Source: CAD feature listing. Evaluate the final solid. Frame: model axes, mm. Face numbers are marked on the shaded views. A direction names the side the tool comes from. Coordinates: 2 decimals unless noted, no trailing zeros. Loops run counter-clockwise (first coordinate to the right, second up) from the corner with the lowest first, then second, coordinate; pieces in that order, holes last. Notation, with made-up numbers: (3.25, 9.25) -> (48.25, 9.25) arc R24 ccw to (48.25, 34.25) -> close; hole circle Ø7 at (-4, -30). An arc over 180 degrees is marked (long way). Answer as a JSON object with one key per item and string values. Group by question number.
Autodesk Inventor part; units mm, degrees
ref_plane "YZ Plane" through (0, 0, 0) normal (1, 0, 0) x (0, 1, 0)
ref_plane "XZ Plane" through (0, 0, 0) normal (0, 1, 0) x (-1, 0, 0)
ref_plane "XY Plane" through (0, 0, 0) normal (0, 0, 1) x (1, 0, 0)
sketch "Sketch4" plane through (0, 0, 0) normal (0, 0, 1) x (1, 0, 0)
  line L0 (0, 0) -> (44.9009, -44.9017) construction
  line L1 (44.9009, -44.9017) -> (89.8017, 0) construction
  line L2 (89.8017, 0) -> (0, 0) construction
  circle A0 centre (0, 0) radius 63.5 construction
  line L3 (40.1856, -49.1667) -> (14.1078, -23.0884)
  line L4 (23.0881, -14.1082) -> (49.166, -40.1866)
  arc A1 (23.0881, -14.1082) -> (14.1078, -23.0884) centre (18.5979, -18.5983) ccw
  arc A2 (56.3508, 29.2718) -> (56.3508, -29.2718) centre (89.8017, 0) ccw
  arc A3 (49.166, -40.1866) -> (56.3508, -29.2718) centre (0, 0) ccw
  arc A4 (56.3508, 29.2718) -> (49.166, 40.1866) centre (0, 0) ccw
  line L5 (49.166, 40.1866) -> (56.3508, 29.2718) construction
  line L6 (56.3508, -29.2718) -> (49.166, -40.1866) construction
  line L7 (0, 0) -> (44.9017, 44.9009) construction
  line L8 (44.9017, 44.9009) -> (0, 89.8017) construction
  line L9 (0, 89.8017) -> (0, 0) construction
  circle A5 centre (0, 0) radius 63.5 construction
  line L10 (49.166, 40.1866) -> (23.0884, 14.1078)
  line L11 (14.1082, 23.0881) -> (40.1866, 49.166)
  arc A6 (14.1082, 23.0881) -> (23.0884, 14.1078) centre (18.5983, 18.5979) ccw
  arc A7 (-29.2718, 56.3508) -> (29.2718, 56.3508) centre (0, 89.8017) ccw
  arc A8 (40.1866, 49.166) -> (29.2718, 56.3508) centre (0, 0) ccw
  arc A9 (-29.2718, 56.3508) -> (-40.1856, 49.1667) centre (0, 0) ccw
  line L12 (-40.1856, 49.1667) -> (-29.2718, 56.3508) construction
  line L13 (29.2718, 56.3508) -> (40.1866, 49.166) construction
  line L14 (0, 0) -> (-44.9008, 44.9017) construction
  line L15 (-44.9008, 44.9017) -> (-89.8017, 0) construction
  line L16 (-89.8017, 0) -> (0, 0) construction
  circle A10 centre (0, 0) radius 63.5 construction
  line L17 (-40.1856, 49.1667) -> (-14.1078, 23.0884)
  line L18 (-23.0881, 14.1082) -> (-49.166, 40.1866)
  arc A11 (-23.0881, 14.1082) -> (-14.1078, 23.0884) centre (-18.5979, 18.5983) ccw
  arc A12 (-56.3508, -29.2718) -> (-56.3508, 29.2718) centre (-89.8017, 0) ccw
  arc A13 (-49.166, 40.1866) -> (-56.3508, 29.2718) centre (0, 0) ccw
  arc A14 (-56.3508, -29.2718) -> (-49.1667, -40.1856) centre (0, 0) ccw
  line L19 (-49.1667, -40.1856) -> (-56.3508, -29.2718) construction
  line L20 (-56.3508, 29.2718) -> (-49.166, 40.1866) construction
  line L21 (0, 0) -> (-44.9017, -44.9008) construction
  line L22 (-44.9017, -44.9008) -> (0, -89.8017) construction
  line L23 (0, -89.8017) -> (0, 0) construction
  circle A15 centre (0, 0) radius 63.5 construction
  line L24 (-49.1667, -40.1856) -> (-23.0884, -14.1078)
  line L25 (-14.1082, -23.0881) -> (-40.1866, -49.166)
  arc A16 (-14.1082, -23.0881) -> (-23.0884, -14.1078) centre (-18.5983, -18.5979) ccw
  arc A17 (29.2718, -56.3508) -> (-29.2718, -56.3508) centre (0, -89.8017) ccw
  arc A18 (-40.1866, -49.166) -> (-29.2718, -56.3508) centre (0, 0) ccw
  arc A19 (29.2718, -56.3508) -> (40.1856, -49.1667) centre (0, 0) ccw
  line L26 (40.1856, -49.1667) -> (29.2718, -56.3508) construction
  line L27 (-29.2718, -56.3508) -> (-40.1866, -49.166) construction
  dimension "d22" = 89.8017
  dimension "d23" = 63.5
  dimension "d27" = 12.7
  dimension "d28" = 37.1983
  dimension "d29" = 44.45
extrude "Extrusion3" add sketch "Sketch4" along normal blind 16.9333
ref_plane "Work Plane1" through (0, 0, 8.4667) normal (0, 0, -1) x (-1, 0, 0)
sketch "Sketch19" plane through (0, 0, 16.9333) normal (0, 0, 1) x (1, 0, 0)
  circle A0 centre (0, 0) radius 8.4667
  dimension "d93" = 16.9333
extrude "Extrusion15" cut sketch "Sketch19" against normal through all
ref_plane "Work Plane5" through (14.1078, -14.1081, 0) normal (0.7071, 0.7071, 0) x (-0.7071, 0.7071, 0)
sketch "Sketch20" plane through (14.1078, -14.1081, 0) normal (0.7071, 0.7071, 0) x (-0.7071, 0.7071, 0)
  line L0 (-6.35, 0) -> (-6.35, 16.9333)
  line L1 (-6.35, 0) -> (-6.35, 16.9333)
  line L2 (-6.35, 16.9333) -> (-82.55, 16.9333)
  line L3 (-40.5924, 16.9333) -> (0.8046, 16.9333)
  line L4 (-82.55, 16.9333) -> (-82.55, 10.5833)
  line L5 (-6.35, 0) -> (-43.23, 0)
  line L6 (-82.55, 0) -> (-6.35, 0) construction
  line L7 (19.9517, 0) -> (19.9517, 76.2)
  line L8 (-6.35, 16.9333) -> (6.35, 16.9333)
  line L9 (6.35, 16.9333) -> (6.35, 0)
  line L10 (6.35, 0) -> (-6.35, 0)
  line L11 (-82.55, 16.9333) -> (-82.55, 10.5833)
  line L12 (-82.55, 10.5833) -> (-6.35, 10.5833)
  line L13 (-6.35, 10.5833) -> (6.35, 10.5833)
  line L14 (-82.55, 10.5833) -> (-82.55, 0) construction
  dimension "d96" = 76.2
  dimension "d97" = 76.2
  dimension "d98" = 12.7
  dimension "d99" = 6.35
revolve "Revolution3" cut sketch "Sketch20" angle 360 about axis through (0, 0, 0) along (0, 0, 1) contours L12 L4 L2 L0 | L0 L3 L8 L9 L13
properties part number "Geneva Driven" material "ABS Plastic"
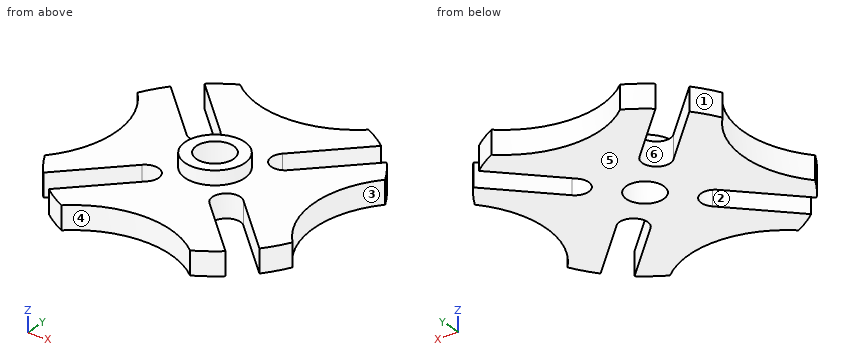
1. Section query D-D on y = -37.5. Return loops of the section in (x, z), then the cut area to 3 significant figures.
2. Reachability of the marked faces 1 and 2 from +Z, -Z, +X, -X, +Y, -Y: full face, straight path, thin tool, end or side. Return the list, or none.
3. Pin query (flat end, axial travel): pin 1 Ø2 at (y, z) = (12, 7.5) entering from +X; pin 2 Ø1 at (y, z) = (-23, 8) entering from +X; pin 3 Ø5 at (y, z) = (11.5, 12.5) entering from -X. Return the tip coordinate at first contact, or that it passes through.
4. Section query B-B on z = 5.75. Return loops of the section in (x, y).
5. Section query A-A on y = 0. Return loops of the section in (x, z).
6. Mould query, pull axis X, two halves, no side actions, for the marked faces 3, 4, 5 and 6. Classes: pulls with the +X half, pulls with the -X half, needs draft (parallel to the pull), parting line crosses it, or undercut.
7. Ray query, L1, parallel to X at y = -38.5, z = 10.5; L2, parallel to X at y = 30, z = 4.5; L3, parallel to Y at x = -26, z = 10.5. Return the intervals inside material, ascending.
Solved:
{
 "1": {"outline": "(-51.24, 0) -> (-46.48, 0) -> (-46.48, 10.58) -> (-51.24, 10.58) -> close; (-28.52, 0) -> (28.52, 0) -> (28.52, 10.58) -> (-28.52, 10.58) -> close; (46.48, 0) -> (51.24, 0) -> (51.24, 10.58) -> (46.48, 10.58) -> close", "area": "705 mm^2"},
 "2": {"face 1": "+Z, -Z, -X, +Y", "face 2": "+Z, -Z"},
 "3": {"pin 1": "x = 47.3", "pin 2": "x = 52.07", "pin 3": "x = -47.33"},
 "4": {"outline": "(-56.35, -29.27) arc R63.5 ccw to (-49.17, -40.19) -> (-23.09, -14.11) arc R6.35 cw to (-14.11, -23.09) -> (-40.19, -49.17) arc R63.49 ccw to (-29.27, -56.35) arc R44.45 cw to (29.27, -56.35) arc R63.5 ccw to (40.19, -49.17) -> (14.11, -23.09) arc R6.35 cw to (23.09, -14.11) -> (49.17, -40.19) arc R63.49 ccw to (56.35, -29.27) arc R44.45 cw to (56.35, 29.27) arc R63.51 ccw to (49.17, 40.19) -> (23.09, 14.11) arc R6.35 cw to (14.11, 23.09) -> (40.19, 49.17) arc R63.49 ccw to (29.27, 56.35) arc R44.45 cw to (-29.27, 56.35) arc R63.5 ccw to (-40.19, 49.17) -> (-14.11, 23.09) arc R6.35 cw to (-23.09, 14.11) -> (-49.17, 40.19) arc R63.49 ccw to (-56.35, 29.27) arc R44.45 cw to start; hole circle Ø16.93 at (0, 0)"},
 "5": {"outline": "(-45.35, 0) -> (-8.47, 0) -> (-8.47, 16.93) -> (-13.6, 16.93) -> (-13.6, 10.58) -> (-45.35, 10.58) -> close; (8.47, 0) -> (45.35, 0) -> (45.35, 10.58) -> (13.6, 10.58) -> (13.6, 16.93) -> (8.47, 16.93) -> close"},
 "6": {"face 3": "pulls with the +X half", "face 4": "undercut", "face 5": "needs draft", "face 6": "undercut"},
 "7": {"L1": "-50.5 to -47.48, -29.52 to 29.52, 47.48 to 50.5", "L2": "-55.97 to -38.98, -21.02 to 21.02, 38.98 to 55.97", "L3": "-53.75 to -34.98, -17.02 to 17.02, 34.98 to 53.75"}
}
